Geometry: final body of the model. Coordinates: model frame, mm. A direction names the side the tool comes from. Round coordinates to 2 decimals unless told otherwise and drop trailing zeros. Order: outer loops, then holes, each group sorted by start corner. A loop starts at its lowest first (then second) coordinate and runs counter-clockwise, first axis right, second up. Notation, with made-up numbers: M 70,77 L 103,77 A29 cw 103,110 Z; hole C -5,11 d6. An arc over 180 degrees is marked long. Put each result on its own line as item: value. Start each with the question number.
1) Section C-C, the plane y = 5.25. Return loops of the section in (x, z), then the cut area to 3 significant figures.
2) Material intervals for probe 1 along X at (y, z) = (0.25, 1); probe 2 along Z at (x, y) = (-13, 1); probe 3 along Z at (x, y) = (-9.95, 5.5), sorted ascending. Write a range as [from, to].
3) Draft query along Z for faces 1 (the cylindrical face through (-3.28, 4.93, -5.02)), 2 (the cylindrical face through (-13.03, 5.07, 10.82)), 3 (the flat face through (-13.912, 4.93, -8.716)). Return one class per face: pulls with the +Z half, pulls with the -Z half, needs draft (parallel to the pull), parting line crosses it, or undercut.
4) Access query for faces 4 (the cylindrical face through (-7.37, 4.93, -11.22)), 5 (the flat face through (-16, 5, -0.75)), 6 (the flat face through (-26.47, -7.4, 16.31)). Directions: +Z, -Z, +X, -X, +Y, -Y. A direction counts if a zero-diameter tool reaches every point of the face in a straight line with its end or side. Return the directions, or none.
5) Section D-D, the plane z = 3. Return loops of the section in (x, y), then the cut area to 3 significant figures.
6) Section A-A, the plane x = -18. Return loops of the section in (y, z), then the cut area to 3 significant figures.
7) Section B-B, the plane x = -3.75. Return loops of the section in (y, z), then the cut area to 3 significant figures.
8) First-contact query: P1, Ø18, axis at x = -10.5, z = 12, coming from the -Y side; P2, Ø4, axis at y = 1.5, z = 18.5, coming from the -X side; P3, Ø2, axis at x = -14.5, y = 7, coming from the -Z side. Flat tips, straight axial feed; report the tip coordinate or a pass-through.
from build123d import *

# Parameters (mm, degrees)
SKETCH1_R                       = 1.55
SKETCH1_R_2                     = 2.45
BOSS_EXTRUDE1_DEPTH             = 10
SKETCH2_W                       = 9.45
SKETCH2_H                       = 1.5
CUT_EXTRUDE1_DEPTH              = 25.542893997
BOSS_EXTRUDE3_DEPTH             = 10
BOSS_EXTRUDE4_DEPTH             = 15
F_3_0MM_CLEARANCE_DOWEL_HOLE2_D = 3.108
F_3_0MM_CLEARANCE_DOWEL_HOLE3_D = 3.108
FILLET2_R                       = 7


with BuildPart() as part:
    # Sketch1 → Boss-Extrude1 (new body)
    with BuildSketch(Plane(origin=(0, 0, 0), x_dir=(1, 0, 0), z_dir=(0, 1, 0))):
        with BuildLine():
            Line((11.25, 2.165063509), (-2.121223771, 9.884943153))
            ThreePointArc((-2.121223771, 9.884943153), (-7.442989886, 11.219511103), (-12.667897108, 9.545411133))
            Line((-12.667897108, 9.545411133), (-15.191606303, 7.863082307))
            ThreePointArc((-15.191606303, 7.863082307), (-19.4, 0), (-15.191606303, -7.863082307))
            Line((-15.191606303, -7.863082307), (-12.667897108, -9.545411133))
            ThreePointArc((-12.667897108, -9.545411133), (-7.442989886, -11.219511103), (-2.121223771, -9.884943153))
            Line((-2.121223771, -9.884943153), (11.25, -2.165063509))
            ThreePointArc((11.25, -2.165063509), (12.5, 0), (11.25, 2.165063509))
        make_face()
        with Locations(Location((7.5, 0, 0), (0, 0, 270))):
            Circle(SKETCH1_R, mode=Mode.SUBTRACT)
        with Locations(Location((-3.75, 6.495190528, 0), (0, 0, 270))):
            Circle(SKETCH1_R, mode=Mode.SUBTRACT)
        with Locations(Location((-9.95, 0, 0), (0, 0, 270))):
            Circle(SKETCH1_R_2, mode=Mode.SUBTRACT)
    extrude(amount=BOSS_EXTRUDE1_DEPTH)

    # Sketch2 → Cut-Extrude1 (cut, through all)
    with BuildSketch(Plane(origin=(0, 10, 0), x_dir=(1, 0, 0), z_dir=(0, 1, 0))):
        with Locations((-14.675, 0)):
            Rectangle(SKETCH2_W, SKETCH2_H)
    extrude(amount=-CUT_EXTRUDE1_DEPTH, mode=Mode.SUBTRACT)

    # Sketch3 → Boss-Extrude3 (add)
    with BuildSketch(Plane.XZ):
        with BuildLine():
            Line((-35.868683143, 22.59247598), (-22.285990587, -0.93343763))
            Line((-22.285990587, -0.93343763), (-19.370191081, 0.75))
            ThreePointArc((-19.370191081, 0.75), (-18.098070975, 4.786589536), (-15.191606303, 7.863082307))
            Line((-15.191606303, 7.863082307), (-12.667897108, 9.545411133))
            Line((-12.667897108, 9.545411133), (-31.538556124, 25.09247598))
            Line((-31.538556124, 25.09247598), (-35.868683143, 22.59247598))
        make_face()
    extrude(amount=-BOSS_EXTRUDE3_DEPTH)

    # Sketch4 → Boss-Extrude4 (add)
    with BuildSketch(Plane(origin=(0, 0, 0), x_dir=(1, 0, 0), z_dir=(0, 1, 0))):
        Polygon((-35.868683143, -22.59247598), (-25.868683143, -5.271967904), (-21.538556124, -7.771967904), (-31.538556124, -25.09247598), align=None)
    extrude(amount=-BOSS_EXTRUDE4_DEPTH)

    # Ø3.0mm Clearance Dowel Hole2 (through all)
    with Locations(Plane(origin=(-12.788556272, 0, -7.383476406), x_dir=(0.5000000000000013, 0, -0.8660254037844379), z_dir=(0.8660254037844379, 0, 0.5000000000000013))):
        with Locations((-22.499999704, -7.5), (-32.499999704, -7.5)):
            Hole(F_3_0MM_CLEARANCE_DOWEL_HOLE2_D / 2)

    # Ø3.0mm Clearance Dowel Hole3 (through all)
    with Locations(Plane(origin=(0, 0, 0), x_dir=(-1, 0, 0), z_dir=(0, -1, 0))):
        with Locations((18.297907491, -9.642957265)):
            Hole(F_3_0MM_CLEARANCE_DOWEL_HOLE3_D / 2)

    # Fillet2
    fillet2_edges = [part.edges().sort_by_distance(p)[0] for p in [
        (-12.667897108, 5, 9.545411133),
    ]]
    fillet(fillet2_edges, radius=FILLET2_R)


solid = part.part
Result sheet:
1. outline: M -35.87,22.59 L -22.29,-0.93 L -19.37,0.75 L -12.28,0.75 A2.45 cw long -12.28,-0.75 L -19.37,-0.75 A9.45 ccw -15.19,-7.86 L -12.67,-9.55 A10 ccw -2.12,-9.88 L 11.25,-2.17 A2.5 ccw 11.25,2.17 L -2.12,9.88 A10 ccw -9.7,10.89 A7 cw -15.95,12.25 L -31.54,25.09 Z; hole C -18.3,9.64 d3.11; hole C -3.75,-6.5 d3.1; hole C 7.5,0 d3.1
1. area: 670 mm2
2. probe 1: x = [-23.4, -12.19], [-7.71, 6.32], [8.68, 12.29]
2. probe 2: z = [-9.32, -0.75], [0.75, 10.81]
2. probe 3: z = [-10.82, -2.45], [2.45, 10.82]
3. face 1: undercut
3. face 2: pulls with the +Z half
3. face 3: pulls with the -Z half
4. face 4: -Z, +Y, -Y
4. face 5: +Y, -Y
4. face 6: +Z, +X, -Y
5. outline: M -24.56,0 L 9.8,0 L 9.8,10 L -24.56,10 Z
5. area: 344 mm2
6. outline: M 0,-4.95 L 10,-4.95 L 10,-0.75 L 0,-0.75 Z; M 0,0.75 L 10,0.75 L 10,8.12 L 0,8.12 Z; M 0,11.17 L 10,11.17 L 10,13.94 L 0,13.94 Z
6. area: 143 mm2
7. outline: M 0,-10.64 L 10,-10.64 L 10,-8.05 L 0,-8.05 Z; M 0,-4.95 L 10,-4.95 L 10,10.64 L 0,10.64 Z
7. area: 182 mm2
8. P1: stops at y = 0
8. P2: stops at x = -34.66
8. P3: stops at z = -8.99
